```python
from build123d import *

# Parameters (mm, degrees)
BOSS_EXTRUDE1_DEPTH = 5.08
SKETCH2_R           = 1.5875
CUT_EXTRUDE1_DEPTH  = 220.530070833
SKETCH3_W           = 5.08
SKETCH3_H           = 20.602222222
CUT_EXTRUDE2_DEPTH  = 220.530070833
CUT_EXTRUDE3_DEPTH  = 220.530070833


with BuildPart() as part:
    # Sketch1 → Boss-Extrude1 (new body)
    with BuildSketch(Plane.XY):
        Polygon((0, 0), (17.78, 0), (17.78, 15.24), (35.56, 15.24), (35.56, 0), (53.34, 0), (53.34, 15.24), (71.12, 15.24), (71.12, 0), (88.9, 0), (88.9, -185.42), (71.12, -185.42), (71.12, -200.66), (53.34, -200.66), (53.34, -185.42), (35.56, -185.42), (35.56, -200.66), (17.78, -200.66), (17.78, -185.42), (0, -185.42), align=None)
    extrude(amount=BOSS_EXTRUDE1_DEPTH)

    # Sketch2 → Cut-Extrude1 (cut, through all)
    with BuildSketch(Plane.XY.offset(5.08)):
        with Locations((21.59, -93.98)):
            Circle(SKETCH2_R)
        with Locations((67.31, -93.98)):
            Circle(SKETCH2_R)
        with Locations((67.31, -160.02)):
            Circle(SKETCH2_R)
        with Locations((21.59, -160.02)):
            Circle(SKETCH2_R)
    extrude(amount=-CUT_EXTRUDE1_DEPTH, mode=Mode.SUBTRACT)

    # Sketch3 → Cut-Extrude2 (cut, through all)
    with BuildSketch(Plane(origin=(0, 0, 0), x_dir=(-1, 0, 0), z_dir=(0, 0, -1))):
        with Locations((-44.45, -154.516666667)):
            Rectangle(SKETCH3_W, SKETCH3_H)
        with Locations((-44.45, -72.107777778)):
            Rectangle(SKETCH3_W, SKETCH3_H)
        with Locations((-44.45, -30.903333333)):
            Rectangle(SKETCH3_W, SKETCH3_H)
        with Locations((-44.45, -113.312222222)):
            Rectangle(SKETCH3_W, SKETCH3_H)
    extrude(amount=-CUT_EXTRUDE2_DEPTH, mode=Mode.SUBTRACT)

    # Sketch4 → Cut-Extrude3 (cut, through all)
    with BuildSketch(Plane(origin=(0, 0, 0), x_dir=(-1, 0, 0), z_dir=(0, 0, -1))):
        Polygon((-88.9, 0), (-76.2, 0), (-76.2, -63.5), (-82.55, -63.5), (-82.55, -114.3), (-88.9, -114.3), (-88.9, -63.5), align=None)
        Polygon((-6.35, -63.5), (-12.7, -63.5), (-12.7, 0), (0, 0), (0, -63.5), (0, -114.3), (-6.35, -114.3), align=None)
    extrude(amount=-CUT_EXTRUDE3_DEPTH, mode=Mode.SUBTRACT)


solid = part.part
```
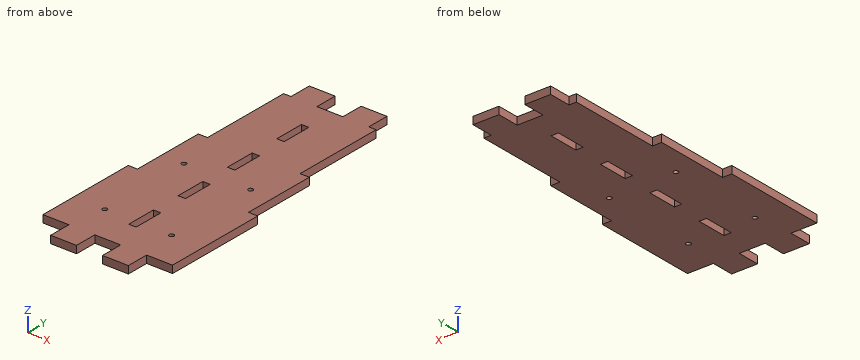
Part model, mm, in its own coordinate system. Give positions to 0.01 mm unless a question says otherwise; leave off trailing zeros. Order: outer loops, then holes, each group sorted by start corner. A loop starts at its lowest first (then second) coordinate and runs counter-clockwise, first axis right, second up. Notation, with made-up numbers: M 41.5,20.25 L 94.5,20.25 A25 cw 94.5,41.25 Z; hole C -23,38 d10. An arc over 180 degrees is marked long. Use a Markdown table: item, result. Add a question column.
(1) Drop flat-ended pins along their axis: P1, Ø1.5, axis at y = -68.5, z = 2, coming from the -X side; P2, Ø2.5, axis at x = 16, z = 2.5, coming from the +Y side; P3, Ø1.5, axis at x = 78, z = 2.5, coming from the +Y side. Give the stop position or say it passes through.
(2) Saw through at C-C, the plane y = -53. Give the cut face in (x, z).
(3) Saw through at B-B, the plane z = 2.05. Give the number of separate pieces and of enclosed holes in the cut face, and give its area (3 significant figures).
(4) Saw through at A-A, the plane y = -109. Give the cut face in (x, z), and give its area (3 significant figures).
(5) Probe line 1 along X through (y, z) = (-93.98, 1.2); line 2 along Y through (x, z) = (67.31, 3.8); line 3 along X through (y, z) = (-160.02, 2.9). List the from-to ranges inside material, lowest first. Write a range as [from, to].
Answer key:
| question | item | result |
|---|---|---|
| 1 | P1 | x = 6.35 |
| 1 | P2 | y = 0 |
| 1 | P3 | y = -63.5 |
| 2 | outline | M 12.7,0 L 76.2,0 L 76.2,5.08 L 12.7,5.08 Z |
| 3 | separate pieces | 1 |
| 3 | enclosed holes | 8 |
| 3 | area | 14,900 mm^2 |
| 4 | outline | M 6.35,0 L 41.91,0 L 41.91,5.08 L 6.35,5.08 Z; M 46.99,0 L 82.55,0 L 82.55,5.08 L 46.99,5.08 Z |
| 4 | area | 361 mm^2 |
| 5 | line 1 | [6.35, 20], [23.18, 65.72], [68.9, 82.55] |
| 5 | line 2 | [-200.66, -161.61], [-158.43, -95.57], [-92.39, 15.24] |
| 5 | line 3 | [0, 20], [23.18, 41.91], [46.99, 65.72], [68.9, 88.9] |
